Print and shaded views of the part. All mm, measured from the part's lowest x, y and z. A direction names the side the tool comes from. Round coordinates to 2 decimals unless told otherwise and drop trailing zeros. Loops run counter-clockwise (first coordinate to the right, second up) from the corner with the lowest first, then second, coordinate; pieces in that order, holes last. Notation, with made-up numbers: (-39.75, 84.25) - (-17.75, 84.25) arc R23 ccw to (-17.75, 114.25) - close; hole circle Ø2 at (17.25, -9). An arc over 180 degrees is marked (long way). Use one line per item in the form item = value.
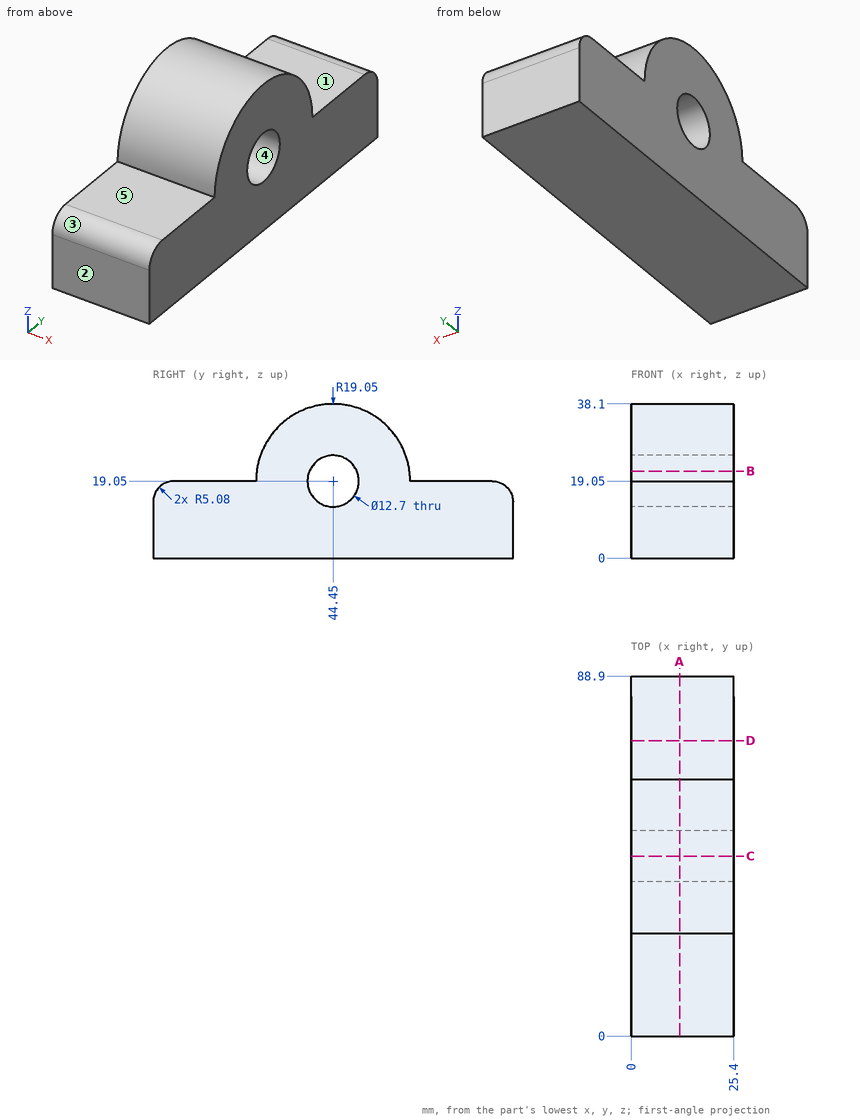
1) Slice it at C-C (y = 44.45). Write the cut outline in (x, z), plus the area to 3 significant figures.
Report:
outline = (0, 0) - (25.4, 0) - (25.4, 12.7) - (0, 12.7) - close; (0, 25.4) - (25.4, 25.4) - (25.4, 38.1) - (0, 38.1) - close
area = 645 mm^2
2) Two-plate mould, pull along Y, no slides. Class the marked faces 3, 4 and 5: +Y half, -Y half, draft (parallel to the pull), parting line (faces both ways), or undercut.
Report:
face_3 = -Y half
face_4 = undercut
face_5 = draft
3) Slice it at B-B (z = 21.5). Write the cut outline in (x, y), plus the area to 3 significant figures.
Report:
outline = (0, 25.56) - (25.4, 25.56) - (25.4, 38.59) - (0, 38.59) - close; (0, 50.31) - (25.4, 50.31) - (25.4, 63.34) - (0, 63.34) - close
area = 662 mm^2
4) Flat gauge pins, fed straight in: pin 1 (10 mm diameter, centred on x = 16, y = 69, fed in from +Z); pin 2 (11.5 mm diameter, centred on y = 44.45, z = 19.05, fed in from +X); pin 3 (12 mm diameter, centred on x = 10, z = 26, fed in from -Y); pin 4 (6 mm diameter, centred on x = 21, z = 30, fed in from +Y). Where does each tip first touch, or does it go through?
Report:
pin_1 = 19.05
pin_2 = through
pin_3 = 25.42
pin_4 = 61.76
5) Slice it at A-A (x = 12). Write the cut outline in (y, z), plus the area to 3 significant figures.
Report:
outline = (0, 0) - (88.9, 0) - (88.9, 13.97) arc R5.08 ccw to (83.82, 19.05) - (63.5, 19.05) arc R19.05 ccw to (25.4, 19.05) - (5.08, 19.05) arc R5.08 ccw to (0, 13.97) - close; hole circle Ø12.7 at (44.45, 19.05)
area = 2,130 mm^2
6) Drill centre lines: probe 1 along Z at (x, y) = (12.75, 44.45); probe 2 along Z at (x, y) = (20.5, 72); probe 3 along Z at (x, y) = (9.75, 32). Where is each one in solid material? Low to high.
Report:
probe_1 = 0 to 12.7, 25.4 to 38.1
probe_2 = 0 to 19.05
probe_3 = 0 to 33.47
7) Tool access for the marked faces 1 and 2: list every direction of +Z, -Z, +X, -X, +Y, -Y with a clear straight run to the whole face (end or side of a thin tool).
Report:
face_1 = +Z, +X, -X, +Y
face_2 = +Z, -Z, +X, -X, -Y
8) Slice it at D-D (y = 73). Write the cut outline in (x, z), plus the area to 3 significant figures.
Report:
outline = (0, 0) - (25.4, 0) - (25.4, 19.05) - (0, 19.05) - close
area = 484 mm^2
